Job drawing, mm, ordinate dimensions from the low corner. One solid piece. Round coordinates to 2 decimals unless told otherwise and drop trailing zeros. Write each loop counter-clockwise with the first axis right and the second up, starting at its lowest first coordinate (ties: lowest second). Pieces come first, ordered by that corner, then holes. Notation, with made-up numbers: (57.25, 68.5) - (108.25, 68.5) arc R10 ccw to (108.25, 84.5) - close; hole circle Ø3 at (-30, 2). An arc over 180 degrees is marked (long way). Write each question's results on one line, items separated by ' | '.
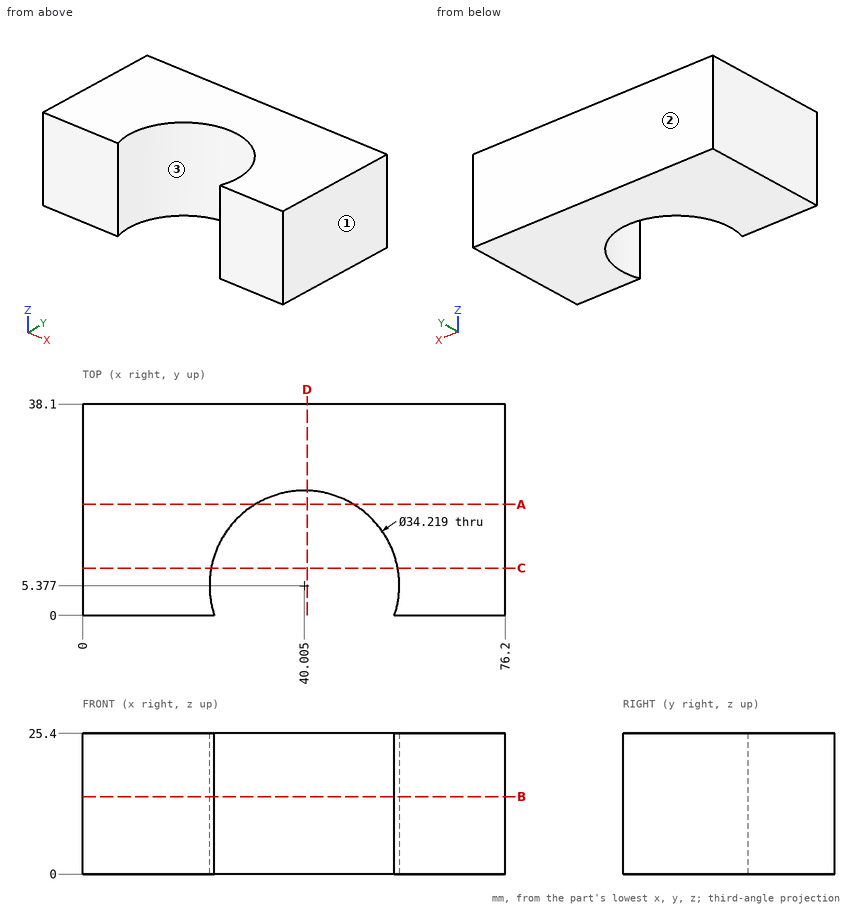
(1) Slice it at D-D, the plane x = 40.5. Write the cut outline in (y, z).
Worked answers:
outline: (22.48, 0) - (38.1, 0) - (38.1, 25.4) - (22.48, 25.4) - close
(2) Slice it at B-B, the plane z = 14. Write the cut outline in (x, y) (1 decimal), and give its area (3 significant figures).
Worked answers:
outline: (0, 0) - (23.8, 0) arc R17.1 cw (long way) to (56.2, 0) - (76.2, 0) - (76.2, 38.1) - (0, 38.1) - close | area: 2,260 mm2
(3) Drill centre lines: probe 1 along X at (y, z) = (12, 21.5); probe 2 along X at (y, z) = (13, 9.25); probe 3 along Y at (x, z) = (46, 17.75). Where is each one in solid material? Low to high. Write a range as [from, to].
Worked answers:
probe 1: x = [0, 24.23], [55.78, 76.2] | probe 2: x = [0, 24.69], [55.32, 76.2] | probe 3: y = [21.4, 38.1]
(4) Two-plate mould, pull along X, no slides. Class the marked faces 1, 2 and 3: released by +X, released by -X, zero draft, split by the parting line, or undercut.
Worked answers:
face 1: released by +X | face 2: zero draft | face 3: undercut
(5) Slice it at C-C, the plane y = 8.5. Write the cut outline in (x, z).
Worked answers:
outline: (0, 0) - (23.18, 0) - (23.18, 25.4) - (0, 25.4) - close; (56.83, 0) - (76.2, 0) - (76.2, 25.4) - (56.83, 25.4) - close
(6) Slice it at A-A, the plane y = 20. Write the cut outline in (x, z).
Worked answers:
outline: (0, 0) - (31.12, 0) - (31.12, 25.4) - (0, 25.4) - close; (48.89, 0) - (76.2, 0) - (76.2, 25.4) - (48.89, 25.4) - close
(7) Flat gauge pin, fed straight in: pin 1 Ø5 at (x, z) = (45, 2.5) entering from -Y. Where does the tip first touch, or does it go through?
Worked answers:
pin 1: stops at y = 20.76
